Design review of the part built by this model. Coordinates are the model's own, in mm. Face numbers are marked on the shaded views. Coordinates: 2 decimals unless noted, no trailing zeros. Write each loop counter-clockwise with the first axis right and the second up, starting at its lowest first coordinate (ties: lowest second). Pieces come first, ordered by that corner, then holes.
Q1. Take a section at C-C (x = 10). Give the boundary of the cut face in (y, z), and give its area (3 significant figures).
Q2. For probe 1 along X at (y, z) = (-1.9, 45); probe 2 along X at (y, z) = (4, 31.5); probe 3 along Y at (x, z) = (-1.25, 37), list the stretches that pass through material, from the lowest coordinate up.
Q3. Take a section at B-B (z = 35). Give the boundary of the cut face in (x, y).
Q4. Insertion check: pin 1 (3.5 mm diameter, centred on x = -10, z = 45, fed in from +Y); pin 2 (4.5 mm diameter, centred on x = 0, z = 15, fed in from +Y). Each pin has a flat end and moves straight along its axis. Give the tip position at first contact, or say it passes through.
Q5. Take a section at D-D (z = 18). Give the boundary of the cut face in (x, y).
Q6. Take a section at A-A (y = 0). Give the boundary of the cut face in (x, z), and give its area (3 significant figures).
Q7. Mouldability with a two-part tool opening along X and no side actions: class the marked faces 1, 2, 3 and 4 as pulls with the +X half, pulls with the -X half, needs draft (parallel to the pull), parting line crosses it, or undercut.
Autodesk Inventor part; units mm, degrees
ref_plane "YZ Plane" through (0, 0, 0) normal (1, 0, 0) x (0, 1, 0)
ref_plane "XZ Plane" through (0, 0, 0) normal (0, 1, 0) x (-1, 0, 0)
ref_plane "XY Plane" through (0, 0, 0) normal (0, 0, 1) x (1, 0, 0)
sketch "Náčrt1" plane through (0, 0, 0) normal (0, 0, 1) x (1, 0, 0)
  line L0 (-14.5, 7.7937) -> (-14.5, -1.7063)
  line L1 (-14.5, -1.7063) -> (14.5, -1.7063)
  line L2 (14.5, -1.7063) -> (14.5, 7.7937)
  line L3 (14.5, 7.7937) -> (15, 7.7937)
  line L4 (15, 7.7937) -> (15, -2.2063)
  line L5 (15, -2.2063) -> (-15, -2.2063)
  line L6 (-15, -2.2063) -> (-15, 7.7937)
  line L7 (-15, 7.7937) -> (-14.5, 7.7937)
  point P0 (0, 0)
  point P1 (14.5, 3.0437)
  point P2 (-14.75, 7.7937)
  point P3 (14.75, 7.7937)
  dimension "d0" = 15
  dimension "d1" = 15
  dimension "d2" = 0.5
  dimension "d3" = 0.5
  dimension "d4" = 0.5
  dimension "d5" = 10
  dimension "d6" = 10
extrude "Vysunutí1" add sketch "Náčrt1" along normal blind 50
sketch "Náčrt2" plane through (15, -2.2063, 0) normal (1, 0, 0) x (0, 0, -1)
  circle A0 centre (-5, 5) radius 2
  line L0 (0, 0) -> (0, 10)
  point P0 (0, 2.2063)
  point P1 (0, 5)
  dimension "d9" = 4
  dimension "d10" = 5
extrude "Vysunutí2" cut sketch "Náčrt2" against normal through all
pattern_linear "Obdélníkové pole1" count 10 spacing 10 along (0, 0, 1) of "Vysunutí2"
sketch "Náčrt3" plane through (-14.5, -1.7063, 0) normal (0, 1, 0) x (1, 0, 0)
  circle A0 centre (4.5, -45) radius 2
  line L0 (29, -50) -> (0, -50)
  line L1 (-0.5, 0) -> (-0.5, -50)
  point P0 (14.5, 0)
  dimension "d16" = 4
  dimension "d17" = 5
  dimension "d18" = 5
extrude "Vysunutí3" cut sketch "Náčrt3" against normal through all
pattern_linear "Obdélníkové pole2" count 10 spacing 10 along (0, 0, -1) count 5 spacing 10 along (1, 0, 0) of "Vysunutí3"
properties part number "1024 cervena"
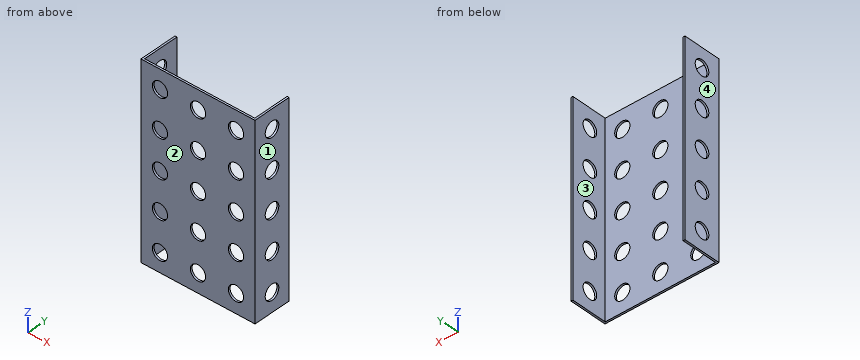
Response:
1. outline: (-2.21, 0) - (-1.71, 0) - (-1.71, 3) - (-2.21, 3) - close; (-2.21, 7) - (-1.71, 7) - (-1.71, 13) - (-2.21, 13) - close; (-2.21, 17) - (-1.71, 17) - (-1.71, 23) - (-2.21, 23) - close; (-2.21, 27) - (-1.71, 27) - (-1.71, 33) - (-2.21, 33) - close; (-2.21, 37) - (-1.71, 37) - (-1.71, 43) - (-2.21, 43) - close; (-2.21, 47) - (-1.71, 47) - (-1.71, 50) - (-2.21, 50) - close
1. area: 15.0 mm2
2. probe 1: x = -15 to -12, -8 to -2, 2 to 8, 12 to 15
2. probe 2: x = -15 to -14.5, 14.5 to 15
2. probe 3: y = -2.21 to -1.71
3. outline: (-15, -2.21) - (-12, -2.21) - (-12, -1.71) - (-14.5, -1.71) - (-14.5, 0.79) - (-15, 0.79) - close; (-15, 4.79) - (-14.5, 4.79) - (-14.5, 7.79) - (-15, 7.79) - close; (-8, -2.21) - (-2, -2.21) - (-2, -1.71) - (-8, -1.71) - close; (2, -2.21) - (8, -2.21) - (8, -1.71) - (2, -1.71) - close; (12, -2.21) - (15, -2.21) - (15, 0.79) - (14.5, 0.79) - (14.5, -1.71) - (12, -1.71) - close; (14.5, 4.79) - (15, 4.79) - (15, 7.79) - (14.5, 7.79) - close
4. pin 1: passes through
4. pin 2: stops at y = -1.71
5. outline: (-15, -2.21) - (15, -2.21) - (15, 7.79) - (14.5, 7.79) - (14.5, -1.71) - (-14.5, -1.71) - (-14.5, 7.79) - (-15, 7.79) - close
6. outline: (-15, 0) - (-14.5, 0) - (-14.5, 50) - (-15, 50) - close; (14.5, 0) - (15, 0) - (15, 50) - (14.5, 50) - close
6. area: 50.0 mm2
7. face 1: pulls with the +X half
7. face 2: needs draft
7. face 3: undercut
7. face 4: pulls with the -X half
